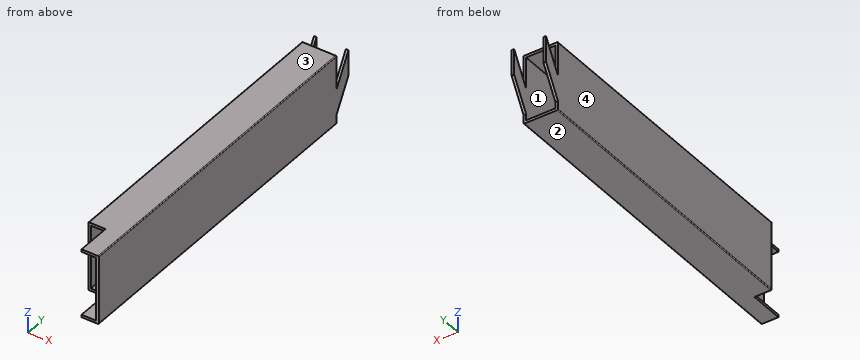
from build123d import *

# Parameters (mm, degrees)
SKETCH1_W           = 17
SKETCH1_H           = 37
BOSS_EXTRUDE1_DEPTH = 208
SKETCH2_W           = 10
SKETCH2_H           = 20
CUT_EXTRUDE1_DEPTH  = 40
CUT_EXTRUDE2_DEPTH  = 40


with BuildPart() as part:
    # Sketch1 → Boss-Extrude1 (new body)
    with BuildSketch(Plane(origin=(0, 0, 0), x_dir=(1, 0, 0), z_dir=(0, 1, 0))):
        with BuildLine():
            Line((0.5, 0), (19.5, 0))
            ThreePointArc((19.5, 0), (19.853553391, 0.146446609), (20, 0.5))
            Line((20, 0.5), (20, 39.5))
            ThreePointArc((20, 39.5), (19.853553391, 39.853553391), (19.5, 40))
            Line((19.5, 40), (0.5, 40))
            ThreePointArc((0.5, 40), (0.146446609, 39.853553391), (0, 39.5))
            Line((0, 39.5), (0, 0.5))
            ThreePointArc((0, 0.5), (0.146446609, 0.146446609), (0.5, 0))
        make_face()
        with Locations((10, 20)):
            Rectangle(SKETCH1_W, SKETCH1_H, mode=Mode.SUBTRACT)
    extrude(amount=BOSS_EXTRUDE1_DEPTH)

    # Sketch2 → Cut-Extrude1 (cut)
    with BuildSketch(Plane.XY):
        with Locations((5, 10)):
            Rectangle(SKETCH2_W, SKETCH2_H)
    extrude(amount=-CUT_EXTRUDE1_DEPTH, mode=Mode.SUBTRACT)

    # Sketch3 → Cut-Extrude2 (cut)
    with BuildSketch(Plane(origin=(0, 0, 0), x_dir=(0, 0, -1), z_dir=(1, 0, 0))):
        Polygon((0, 208), (0, 198), (19.820508076, 198), (2.5, 208), align=None)
        Polygon((17.5, 208), (34.820508076, 198), (40, 198), (40, 208), align=None)
    extrude(amount=CUT_EXTRUDE2_DEPTH, mode=Mode.SUBTRACT)


solid = part.part
Input: part model. Units: mm. Frame: model coordinates. Face numbers are marked on the shaded views. Coordinates: 2 decimals unless noted, no trailing zeros. Order: outer loops, then holes, each group sorted by start corner. A loop starts at its lowest first (then second) coordinate and runs counter-clockwise, first axis right, second up. Notation, with made-up numbers: M 59.25,52 L 109.25,52 A31 cw 109.25,76 Z; hole C 87,63 d6. An arc over 180 degrees is marked long. Answer in a Markdown table with one row per item.
(1) Section query C-C, the plane y = 145. Output: boundary loops of the cut face in (x, z).
Numbers:
| item | result |
|---|---|
| outline | M 0,-39.5 A0.5 ccw 0.5,-40 L 19.5,-40 A0.5 ccw 20,-39.5 L 20,-0.5 A0.5 ccw 19.5,0 L 0.5,0 A0.5 ccw 0,-0.5 Z; hole M 1.5,-38.5 L 18.5,-38.5 L 18.5,-1.5 L 1.5,-1.5 Z |
(2) Material intervals for line 1 (X direction, y = 65, z = -36); line 2 (Z direction, x = 9, y = 139), sorted ascending. Write a range as [from, to].
Numbers:
| item | result |
|---|---|
| line 1 | x = [0, 1.5], [18.5, 20] |
| line 2 | z = [-40, -38.5], [-1.5, 0] |
(3) Draft query along Z for the marked faces 1, 2, 3 and 4. Return one class per face: pulls with the +Z half, pulls with the -Z half, needs draft (parallel to the pull), parting line crosses it, or undercut.
Numbers:
| item | result |
|---|---|
| face 1 | undercut |
| face 2 | pulls with the -Z half |
| face 3 | pulls with the +Z half |
| face 4 | needs draft |
(4) Contact query for flat-ended pins moving along their axis: pin 1 Ø1.2 at (y, z) = (9, -39) entering from -X; pin 2 Ø12 at (x, z) = (17, -25) entering from +Y; pin 3 Ø8 at (x, z) = (18, -35.5) entering from +Y. Output: stop coordinate, or through.
Numbers:
| item | result |
|---|---|
| pin 1 | stops at x = 10 |
| pin 2 | stops at y = 207.02 |
| pin 3 | stops at y = 199.9 |
(5) Section query B-B, the plane z = -13.5. Output: boundary loops of the cut face in (x, y), plus the area to 3 significant figures.
Numbers:
| item | result |
|---|---|
| outline | M 0,20 L 1.5,20 L 1.5,198 L 0,198 Z; M 0,201.65 L 1.5,201.65 L 1.5,208 L 0,208 Z; M 18.5,0 L 20,0 L 20,198 L 18.5,198 Z; M 18.5,201.65 L 20,201.65 L 20,208 L 18.5,208 Z |
| area | 583 mm^2 |
(6) Section query A-A, the plane x = 5.75. Output: boundary loops of the cut face in (y, z), plus the area to 3 significant figures.
Numbers:
| item | result |
|---|---|
| outline | M 20,-40 L 198,-40 L 198,-38.5 L 20,-38.5 Z; M 20,-1.5 L 198,-1.5 L 198,0 L 20,0 Z |
| area | 534 mm^2 |
(7) Section query D-D, the plane z = -22. Output: boundary loops of the cut face in (x, y).
Numbers:
| item | result |
|---|---|
| outline | M 0,20 L 1.5,20 L 1.5,205.4 L 0,205.4 Z; M 18.5,0 L 20,0 L 20,205.4 L 18.5,205.4 Z |
